```python
from build123d import *

# Parameters (mm, degrees)
SKETCH1_W                    = 705
SKETCH1_H                    = 50
BOSS_EXTRUDE1_DEPTH          = 2
CONVERT_SOLID1_OUTLINE_W     = 705
CONVERT_SOLID1_OUTLINE_H     = 50
CONVERT_SOLID1_DEPTH         = 0.5
EDGE_FLANGE1_STRIP_W         = 10
EDGE_FLANGE1_STRIP_H         = 1.5
EDGE_FLANGE1_STRIP_CUT_DEPTH = 705
EDGE_FLANGE1_DEPTH           = 705


# Read off the part's stored shape, not the designer's step: Convert-Solid1
# Sheet-metal steps are written as plain solids
with BuildPart() as part:
    # Sketch1 → Boss-Extrude1 (new body)
    with BuildSketch(Plane(origin=(0, 0, 0), x_dir=(1, 0, 0), z_dir=(0, 1, 0))):
        with Locations((-352.5, 25)):
            Rectangle(SKETCH1_W, SKETCH1_H)
    extrude(amount=BOSS_EXTRUDE1_DEPTH)

    # Convert-Solid1 outline → Convert-Solid1 (cut)
    with BuildSketch(Plane(origin=(0, 0, 0), x_dir=(1, 0, 0), z_dir=(0, 1, 0))):
        with Locations((-352.5, 25)):
            Rectangle(CONVERT_SOLID1_OUTLINE_W, CONVERT_SOLID1_OUTLINE_H)
    extrude(amount=CONVERT_SOLID1_DEPTH, mode=Mode.SUBTRACT)

    # Edge-Flange1 strip (across the edge) → Edge-Flange1 strip cut (cut)
    with BuildSketch(Plane(origin=(-705, 2, 0), x_dir=(0, 0, -1), z_dir=(1, 0, 0))):
        with Locations((-3, -0.75)):
            Rectangle(EDGE_FLANGE1_STRIP_W, EDGE_FLANGE1_STRIP_H)
    extrude(amount=EDGE_FLANGE1_STRIP_CUT_DEPTH, mode=Mode.SUBTRACT)

    # Edge-Flange1 section (across the edge) → Edge-Flange1 (add)
    with BuildSketch(Plane(origin=(-705, 2, 0), x_dir=(0, 0, -1), z_dir=(1, 0, 0))):
        with BuildLine():
            Line((-1.5, 2), (-1.5, 48.5))
            Line((-1.5, 48.5), (0, 48.5))
            Line((0, 48.5), (0, 2))
            ThreePointArc((0, 2), (0.585786438, 0.585786438), (2, 0))
            Line((2, 0), (2, -1.5))
            ThreePointArc((2, -1.5), (-0.474873734, -0.474873734), (-1.5, 2))
        make_face()
    extrude(amount=EDGE_FLANGE1_DEPTH)


solid = part.part
```
Geometry: final body of the model. Coordinates: model frame, mm. A direction names the side the tool comes from. Coordinates: 2 decimals unless noted, no trailing zeros. Order: outer loops, then holes, each group sorted by start corner. A loop starts at its lowest first (then second) coordinate and runs counter-clockwise, first axis right, second up.
Item 1: Section query C-C (y = 28.5). Output: boundary loops of the cut face in (x, z).
Answer:
outline: (-705, 0) - (0, 0) - (0, 1.5) - (-705, 1.5) - close
Item 2: Material intervals for line 1 along Z through (x, y) = (-256, 16.5); line 2 along Y through (x, z) = (-315, -27), sorted ascending.
Answer:
line 1: z = 0 to 1.5
line 2: y = 0.5 to 2
Item 3: Section query B-B (z = -43). Output: boundary loops of the cut face in (x, y).
Answer:
outline: (-705, 0.5) - (0, 0.5) - (0, 2) - (-705, 2) - close
Item 4: Contact query for flat-ended pins moving along their axis: P1, Ø1, axis at x = -144.5, y = 43.5, coming from the -Z side; P2, Ø24, axis at x = -265.5, z = -37, coming from the +Y side. Output: stop coordinate, or through.
Answer:
P1: stops at z = 0
P2: stops at y = 2
Item 5: Section query A-A (x = -388). Output: boundary loops of the cut face in (y, z), then the cut area to 3 significant figures.
Answer:
outline: (0.5, -50) - (2, -50) - (2, -2) arc R2 cw to (4, 0) - (50.5, 0) - (50.5, 1.5) - (4, 1.5) arc R3.5 ccw to (0.5, -2) - close
area: 148 mm2
Item 6: Access query for faces 1 (the face through (-357, 28, 0)), 2 (the face through (-357, 0.5, -26)). Directions: +Z, -Z, +X, -X, +Y, -Y. A direction counts if a zero-diameter tool reaches every point of the face in a straight line with its end or side. Return the directions, or none.
Answer:
face 1: -Z, +X, -X, +Y
face 2: +Z, -Z, +X, -X, -Y
